Input: part model. Units: mm. Frame: model coordinates. Face numbers are marked on the shaded views. A direction names the side the tool comes from. Coordinates: 2 decimals unless noted, no trailing zeros. Loops run counter-clockwise (first coordinate to the right, second up) from the corner with the lowest first, then second, coordinate; pieces in that order, holes last. Notation, with made-up numbers: M 27,55 L 32,55 A11 ccw 32,65 Z; hole C 78,23.25 d8. An arc over 180 degrees is marked long. Use a Markdown table: item, result. Add a question column.
1. Set-up query: the marked faces 1 and 2. Return all of +Z, -Z, +X, -X, +Y, -Y with unobstructed straight access to the full face (end or side cutting, diameter ignored); none if empty.
2. Pin query (flat end, axial travel): pin 1 (8.5 mm diameter, centred on x = -24, y = 22, fed in from +Z); pin 2 (4 mm diameter, centred on x = -83.5, y = 12.5, fed in from -Z); pin 3 (4 mm diameter, centred on y = -7.5, z = -10.5, fed in from -X). Return the tip coordinate at first contact, or that it passes through.
3. Line query: L1, parallel to Y at x = 0, z = 2.5; L2, parallel to Y at x = -63.5, z = 48; L3, parallel to X at y = -6.5, z = 53. Output: solid intervals per line, ascending. Write a range as [from, to].
4. Section A-A on z = -7.5. Output: boundary loops of the cut face in (x, y).
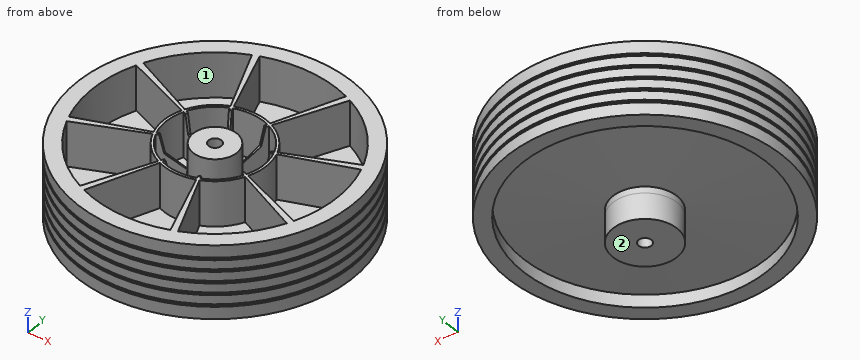
```python
from build123d import *

# Parameters (mm, degrees)
SKETCH1_R           = 107
BOSS_EXTRUDE1_DEPTH = 57
SKETCH3_W           = 2
SKETCH3_H           = 2.636408112
SKETCH7_R           = 25
BOSS_EXTRUDE2_DEPTH = 20
CUT_EXTRUDE1_START  = -35
CUT_EXTRUDE1_DEPTH  = 35
CIRPATTERN5_COUNT   = 8
SKETCH11_R          = 5
CUT_EXTRUDE2_DEPTH  = 170.785158362


with BuildPart() as part:
    # Sketch1 → Boss-Extrude1 (new body)
    with BuildSketch(Plane.XY):
        with Locations(Location((0, 0, 0), (0, 0, 180))):
            Circle(SKETCH1_R)
    extrude(amount=BOSS_EXTRUDE1_DEPTH)

    # Sketch3 → Cut-Revolve3 (revolve, cut)
    with BuildSketch(Plane(origin=(0, 0, 0), x_dir=(0, 0, -1), z_dir=(1, 0, 0)), mode=Mode.PRIVATE) as cut_revolve3_sk:
        with Locations((-46.5, 107.318204056)):
            Rectangle(SKETCH3_W, SKETCH3_H)
        with Locations((-37.5, 107.318204056)):
            Rectangle(SKETCH3_W, SKETCH3_H)
        with Locations((-28.5, 107.318204056)):
            Rectangle(SKETCH3_W, SKETCH3_H)
        with Locations((-19.5, 107.318204056)):
            Rectangle(SKETCH3_W, SKETCH3_H)
        with Locations((-10.5, 107.318204056)):
            Rectangle(SKETCH3_W, SKETCH3_H)
    revolve(cut_revolve3_sk.sketch.rotate(Axis((0, 0, 0), (0, 0, 1)), 90), axis=Axis((0, 0, 0), (0, 0, 1)), mode=Mode.SUBTRACT)

    # Sketch6 → Cut-Revolve4 (revolve, cut)
    with BuildSketch(Plane(origin=(0, 0, 0), x_dir=(0, 0, -1), z_dir=(1, 0, 0)), mode=Mode.PRIVATE) as cut_revolve4_sk:
        Polygon((5, 95), (5, 25), (-5, 25), (-10, 95), align=None)
    revolve(cut_revolve4_sk.sketch.rotate(Axis((0, 0, -20.482166518), (0, 0, 1)), 270), axis=Axis((0, 0, -20.482166518), (0, 0, 1)), mode=Mode.SUBTRACT)

    # Sketch7 → Boss-Extrude2 (add)
    with BuildSketch(Plane(origin=(0, 0, 0), x_dir=(-1, 0, 0), z_dir=(0, 0, -1))):
        Circle(SKETCH7_R)
    extrude(amount=BOSS_EXTRUDE2_DEPTH)

    # Sketch8 → Cut-Extrude1 (cut)
    with BuildSketch(Plane.XY.offset(57).offset(CUT_EXTRUDE1_START)):
        with BuildLine():
            Line((14.334717982, 37.34321706), (34.044955207, 88.690140517))
            ThreePointArc((34.044955207, 88.690140517), (0, 95), (-34.044955207, 88.690140517))
            Line((-34.044955207, 88.690140517), (-14.334717982, 37.34321706))
            ThreePointArc((-14.334717982, 37.34321706), (0, 40), (14.334717982, 37.34321706))
        make_face()
        with BuildLine():
            Line((-13.617982083, 35.476056207), (-6.271439117, 16.337657464))
            ThreePointArc((-6.271439117, 16.337657464), (0, 17.5), (6.271439117, 16.337657464))
            Line((6.271439117, 16.337657464), (13.617982083, 35.476056207))
            ThreePointArc((13.617982083, 35.476056207), (0, 38), (-13.617982083, 35.476056207))
        make_face()
    cut_extrude1 = extrude(amount=CUT_EXTRUDE1_DEPTH, mode=Mode.SUBTRACT)

    # CirPattern5: Cut-Extrude1 ×8 about axis
    cirpattern5_axis = Axis((0, 0, 0), (0, 0, 1))
    for i in range(1, CIRPATTERN5_COUNT):
        add(cut_extrude1.rotate(cirpattern5_axis, i * 360 / CIRPATTERN5_COUNT), mode=Mode.SUBTRACT)

    # Sketch10 → Cut-Revolve5 (revolve, cut)
    with BuildSketch(Plane(origin=(0, 0, 0), x_dir=(0, 0, -1), z_dir=(1, 0, 0)), mode=Mode.PRIVATE) as cut_revolve5_sk:
        Polygon((-58, 35.987045509), (-43, 32.476056207), (-33, 16.987045509), (-58, 16.987045509), align=None)
    revolve(cut_revolve5_sk.sketch.rotate(Axis((0, 0, 0), (0, 0, 1)), 90), axis=Axis((0, 0, 0), (0, 0, 1)), mode=Mode.SUBTRACT)

    # Sketch11 → Cut-Extrude2 (cut, through all)
    with BuildSketch(Plane.XY.offset(57)):
        Circle(SKETCH11_R)
    extrude(amount=-CUT_EXTRUDE2_DEPTH, mode=Mode.SUBTRACT)


solid = part.part
```
Answers below:
| question | item | result |
|---|---|---|
| 1 | face 1 | +Z |
| 1 | face 2 | -Z, +X, -X, +Y, -Y |
| 2 | pin 1 | stops at z = 22 |
| 2 | pin 2 | stops at z = 9.1 |
| 2 | pin 3 | stops at x = -24.39 |
| 3 | L1 | y = [-107, -95], [-25, -5], [5, 25], [95, 107] |
| 3 | L2 | y = [-86.12, -70.66], [-28.27, -24.38], [24.38, 28.27], [70.66, 86.12] |
| 3 | L3 | x = [-106.8, -94.78], [-39.47, -37.44], [-15.69, 15.69], [37.44, 39.47], [94.78, 106.8] |
| 4 | outline | C 0,0 d50; hole C 0,0 d10 |
